Verification items for the finished model (mm, model axes). Round coordinates to 2 decimals unless told otherwise and drop trailing zeros. Loops run counter-clockwise (first coordinate to the right, second up) from the corner with the lowest first, then second, coordinate; pieces in that order, holes last. Notation, with made-up numbers: M 8,-25 L 31,-25 A28 cw 31,-1 Z; hole C 25.25,7 d5. An arc over 180 degrees is marked long. Answer as CSV lines item,"result".
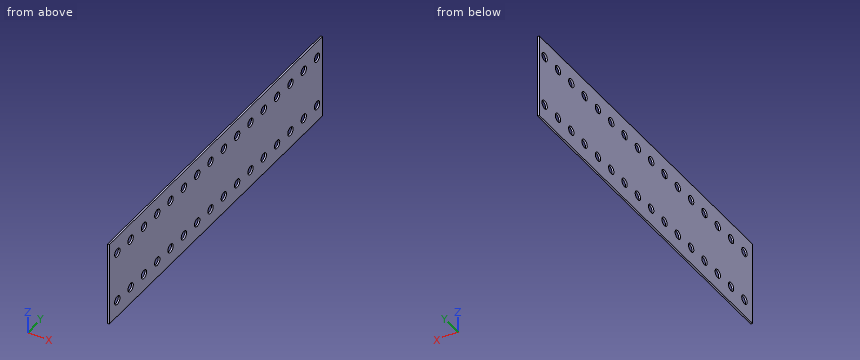
Autodesk Inventor part; units mm, degrees
ref_plane "YZ Plane" through (0, 0, 0) normal (1, 0, 0) x (0, 1, 0)
ref_plane "XZ Plane" through (0, 0, 0) normal (0, 1, 0) x (-1, 0, 0)
ref_plane "XY Plane" through (0, 0, 0) normal (0, 0, 1) x (1, 0, 0)
ref_plane "Work Plane1" through (0, 0, 0) normal (0, 0, 1) x (1, 0, 0)
sketch "Sketch1" plane through (0, 0, 0) normal (0, 0, 1) x (1, 0, 0)
  arc A0 (3437.5, 230) -> (3437.5, 220) centre (3437.5, 225) ccw
  line L0 (3437.5, 230) -> (3452.5, 230)
  arc A1 (3452.5, 220) -> (3452.5, 230) centre (3452.5, 225) ccw
  line L1 (3452.5, 220) -> (3437.5, 220)
  arc A2 (2192.5, 230) -> (2192.5, 220) centre (2192.5, 225) ccw
  line L2 (2192.5, 230) -> (2207.5, 230)
  arc A3 (2207.5, 220) -> (2207.5, 230) centre (2207.5, 225) ccw
  line L3 (2207.5, 220) -> (2192.5, 220)
  arc A4 (942.5, 230) -> (942.5, 220) centre (942.5, 225) ccw
  line L4 (942.5, 230) -> (957.5, 230)
  arc A5 (957.5, 220) -> (957.5, 230) centre (957.5, 225) ccw
  line L5 (957.5, 220) -> (942.5, 220)
  arc A6 (-7.5, 230) -> (-7.5, 220) centre (-7.5, 225) ccw
  line L6 (-7.5, 230) -> (7.5, 230)
  arc A7 (7.5, 220) -> (7.5, 230) centre (7.5, 225) ccw
  line L7 (7.5, 220) -> (-7.5, 220)
  arc A8 (-7.5, -220) -> (-7.5, -230) centre (-7.5, -225) ccw
  line L8 (-7.5, -220) -> (7.5, -220)
  arc A9 (7.5, -230) -> (7.5, -220) centre (7.5, -225) ccw
  line L9 (7.5, -230) -> (-7.5, -230)
  arc A10 (942.5, -220) -> (942.5, -230) centre (942.5, -225) ccw
  line L10 (942.5, -220) -> (957.5, -220)
  arc A11 (957.5, -230) -> (957.5, -220) centre (957.5, -225) ccw
  line L11 (957.5, -230) -> (942.5, -230)
  arc A12 (2192.5, -220) -> (2192.5, -230) centre (2192.5, -225) ccw
  line L12 (2192.5, -220) -> (2207.5, -220)
  arc A13 (2207.5, -230) -> (2207.5, -220) centre (2207.5, -225) ccw
  line L13 (2207.5, -230) -> (2192.5, -230)
  arc A14 (3437.5, -220) -> (3437.5, -230) centre (3437.5, -225) ccw
  line L14 (3437.5, -220) -> (3452.5, -220)
  arc A15 (3452.5, -230) -> (3452.5, -220) centre (3452.5, -225) ccw
  line L15 (3452.5, -230) -> (3437.5, -230)
  line L16 (22.5, -250) -> (22.5, -200)
  line L17 (22.5, -200) -> (927.5, -200)
  line L18 (927.5, -200) -> (927.5, -250)
  line L19 (927.5, -250) -> (972.5, -250)
  line L20 (972.5, -250) -> (972.5, -200)
  line L21 (972.5, -200) -> (2177.5, -200)
  line L22 (2177.5, -200) -> (2177.5, -250)
  line L23 (2177.5, -250) -> (2222.5, -250)
  line L24 (2222.5, -250) -> (2222.5, -200)
  line L25 (2222.5, -200) -> (3422.5, -200)
  line L26 (3422.5, -200) -> (3422.5, -250)
  line L27 (3422.5, -250) -> (3467.5, -250)
  line L28 (3467.5, -250) -> (3467.5, 250)
  line L29 (3467.5, 250) -> (3422.5, 250)
  line L30 (3422.5, 250) -> (3422.5, 200)
  line L31 (3422.5, 200) -> (2222.5, 200)
  line L32 (2222.5, 200) -> (2222.5, 250)
  line L33 (2222.5, 250) -> (2177.5, 250)
  line L34 (2177.5, 250) -> (2177.5, 200)
  line L35 (2177.5, 200) -> (972.5, 200)
  line L36 (972.5, 200) -> (972.5, 250)
  line L37 (972.5, 250) -> (927.5, 250)
  line L38 (927.5, 250) -> (927.5, 200)
  line L39 (927.5, 200) -> (22.5, 200)
  line L40 (22.5, 200) -> (22.5, 250)
  line L41 (22.5, 250) -> (-22.5, 250)
  line L42 (-22.5, 250) -> (-22.5, -250)
  line L43 (-22.5, -250) -> (22.5, -250)
  line L44 (22.5, 200) -> (24.5, 200)
  line L45 (24.5, 200) -> (24.5, -200)
  line L46 (24.5, -200) -> (22.5, -200)
  line L47 (22.5, -200) -> (22.5, 200)
  point P0 (0, 0)
  dimension "d0" = 2
extrude "Extrusion1" add sketch "Sketch1" along normal blind 100 contours L47 L39 L45 L17
sketch "Sketch2" plane through (22.5, -200, 0) normal (-1, 0, 0) x (0, 0, 1)
  line L0 (0, 400) -> (0, 0)
  line L1 (0, 0) -> (100, 0)
  line L2 (100, 400) -> (100, 0)
  line L3 (0, 400) -> (100, 400)
  line L4 (50, 400) -> (50, 0) construction
  line L5 (0, 0) -> (100, 0) construction
  line L6 (0, 200) -> (100, 200) construction
  circle A0 centre (80, 390) radius 5
  dimension "d6" = 10
  dimension "d7" = 20
  dimension "d8" = 10
extrude "Extrusion2" cut sketch "Sketch2" against normal blind 400 contours A0
pattern_linear "Rectangular Pattern1" count 2 spacing 60 along (0, 0, -1) count 16 spacing 25 along (0, -1, 0) of "Extrusion2"
properties part number "Cover Plate"
1) Section check A-A (y = 140). Record the cut outline in (x, z), plus the area to 3 significant figures.
Here are the results:
outline,"M 22.5,0 L 24.5,0 L 24.5,15 L 22.5,15 Z; M 22.5,25 L 24.5,25 L 24.5,75 L 22.5,75 Z; M 22.5,85 L 24.5,85 L 24.5,100 L 22.5,100 Z"
area,"160 mm^2"
2) Go/stop test with a flat-tipped pin: pin 1 (9 mm diameter, centred on y = -35, z = 80, fed in from -X). Record where the tip stops, or that it passes through.
Here are the results:
pin 1,"passes through"
3) Section check B-B (z = 20). State how many separate pieces and enclosed holes the cut face has, plus the area to 3 significant figures.
Here are the results:
separate pieces,"17"
enclosed holes,"0"
area,"480 mm^2"
4) Material ranges on probe 1 along Z at (x, y) = (23.35, 114.5); probe 2 along Z at (x, y) = (22.85, 69.5), recorded low to high.
Here are the results:
probe 1,"z = 0 to 15.03, 24.97 to 75.03, 84.97 to 100"
probe 2,"z = 0 to 17.82, 22.18 to 77.82, 82.18 to 100"
